from build123d import *

# Parameters (mm, degrees)
SKETCH2_R           = 6
BOSS_EXTRUDE2_DEPTH = 36


with BuildPart() as part:
    # Sketch2 → Boss-Extrude2 (new body)
    with BuildSketch(Plane.XY):
        with BuildLine():
            Line((46, 2), (8, 2))
            Line((8, 2), (8, 8))
            Line((8, 8), (5.656854249, 5.656854249))
            ThreePointArc((5.656854249, 5.656854249), (-7.39103626, -3.061467459), (8, 0))
            Line((8, 0), (44, 0))
            ThreePointArc((44, 0), (45.414213562, 0.585786438), (46, 2))
        make_face()
        Circle(SKETCH2_R, mode=Mode.SUBTRACT)
    extrude(amount=BOSS_EXTRUDE2_DEPTH)


solid = part.part
The model under review builds one solid part; all positions refer to its coordinate system, in mm. A direction names the side the tool comes from. Give positions to 0.01 mm unless a question says otherwise; leave off trailing zeros. Write each loop counter-clockwise with the first axis right and the second up, starting at its lowest first coordinate (ties: lowest second). Pieces come first, ordered by that corner, then holes.
1. Add section A-A, the plane x = 0. Write out the cut boundary in (y, z).
2. Wall thickness on L1, parallel to Y at x = 0, z = 16; L2, parallel to X at y = 2.5, z = 24; L3, parallel to Y at x = 1.5, z = 6.5: over which ranges is each line inside the solid? List them lowest first.
3. Tool access review of faces 1 (the flat face through (27, 2, 18)), 2 (the cylindrical face through (-6, 0, 18)), 3 (the flat face through (26, 0, 18)): name each direction out of +Z, -Z, +X, -X, +Y, -Y from which nothing blocks a thin tool from reaching the whole face with its end or side.
4. For P1, Ø7, axis at x = 0, y = 0, coming from the -Z side; P2, Ø3, axis at y = -6, z = 27.5, coming from the +X side; P3, Ø3, axis at y = -6.5, z = 9, coming from the +X side (3 decimals); P4, Ø4, axis at x = 34, z = 24, coming from the -Y side, all flat-tipped, find the tip position at first contact; note any pin that passes through.
5. Add section C-C, the plane y = -2. Write out the cut boundary in (x, z).
6. Add section B-B, the plane z = 18.5. Write out the cut boundary in (x, y).
7. Draft analysis for pull direction X (two halves, no side actions). For faces 4 (the flat face through (13, 1, 0)), 5 (the flat face through (7, 7, 18)), 6 (the cylindrical face through (45.4, 0.57, 17.75)), state which applies: +X half, -X half, draft (parallel to the pull), parting line (faces both ways), or undercut.
8. Add section D-D, the plane x = 37. Write out the cut boundary in (y, z), plus the area to 3 significant figures.
Worked answers:
1. outline: (-8, 0) - (-6, 0) - (-6, 36) - (-8, 36) - close; (6, 0) - (8, 0) - (8, 36) - (6, 36) - close
2. L1: y = -8 to -6, 6 to 8
2. L2: x = -7.6 to -5.45, 5.45 to 8
2. L3: y = -7.86 to -5.81, 5.81 to 7.86
3. face 1: +Z, -Z, +X, +Y
3. face 2: +Z, -Z
3. face 3: +Z, -Z, +X, -Y
4. P1: passes through
4. P2: stops at x = 6.61
4. P3: stops at x = 6.245
4. P4: stops at y = 0
5. outline: (-7.75, 0) - (-5.66, 0) - (-5.66, 36) - (-7.75, 36) - close; (5.66, 0) - (7.75, 0) - (7.75, 36) - (5.66, 36) - close
6. outline: (5.66, 5.66) arc R8 ccw (long way) to (8, 0) - (44, 0) arc R2 ccw to (46, 2) - (8, 2) - (8, 8) - close; hole circle Ø12 at (0, 0)
7. face 4: draft
7. face 5: undercut
7. face 6: +X half
8. outline: (0, 0) - (2, 0) - (2, 36) - (0, 36) - close
8. area: 72.0 mm2
